```python
from build123d import *

# Parameters (mm, degrees)
SKETCH1_R           = 0.75
SKETCH1_R_2         = 0.5
BOSS_EXTRUDE1_DEPTH = 2


with BuildPart() as part:
    # Sketch1 → Boss-Extrude1 (new body)
    with BuildSketch(Plane.XY):
        with BuildLine():
            Line((0, 6), (0, 15))
            Line((0, 15), (4, 15))
            Line((4, 15), (4, 17))
            Line((4, 17), (0, 17))
            Line((0, 17), (0, 20.3))
            ThreePointArc((0, 20.3), (1.464466094, 23.835533906), (5, 25.3))
            Line((5, 25.3), (11.2, 25.3))
            ThreePointArc((11.2, 25.3), (14.735533906, 23.835533906), (16.2, 20.3))
            Line((16.2, 20.3), (16.2, 17))
            Line((16.2, 17), (12.2, 17))
            Line((12.2, 17), (12.2, 15))
            Line((12.2, 15), (16.2, 15))
            Line((16.2, 15), (16.2, 6))
            Line((16.2, 6), (12.2, 6))
            Line((12.2, 6), (12.2, 4))
            Line((12.2, 4), (16.2, 4))
            Line((16.2, 4), (16.2, 2))
            ThreePointArc((16.2, 2), (15.614213562, 0.585786438), (14.2, 0))
            Line((14.2, 0), (2, 0))
            ThreePointArc((2, 0), (0.585786438, 0.585786438), (0, 2))
            Line((0, 2), (0, 4))
            Line((0, 4), (4, 4))
            Line((4, 4), (4, 6))
            Line((4, 6), (0, 6))
        make_face()
        with Locations(Location((6, 12.5, 0), (0, 0, 180))):
            Circle(SKETCH1_R, mode=Mode.SUBTRACT)
        with Locations(Location((10.2, 12.5, 0), (0, 0, 180))):
            Circle(SKETCH1_R, mode=Mode.SUBTRACT)
        with Locations(Location((2.75, 19, 0), (0, 0, 180))):
            Circle(SKETCH1_R, mode=Mode.SUBTRACT)
        with Locations(Location((13.45, 19, 0), (0, 0, 180))):
            Circle(SKETCH1_R, mode=Mode.SUBTRACT)
        with Locations((10.2, 8.5)):
            Circle(SKETCH1_R, mode=Mode.SUBTRACT)
        with Locations((6, 8.5)):
            Circle(SKETCH1_R, mode=Mode.SUBTRACT)
        with Locations((3, 22.3)):
            Circle(SKETCH1_R_2, mode=Mode.SUBTRACT)
        with Locations((13.2, 22.3)):
            Circle(SKETCH1_R_2, mode=Mode.SUBTRACT)
        with Locations((13.45, 2)):
            Circle(SKETCH1_R, mode=Mode.SUBTRACT)
        with Locations((2.75, 2)):
            Circle(SKETCH1_R, mode=Mode.SUBTRACT)
    extrude(amount=BOSS_EXTRUDE1_DEPTH)


solid = part.part
```
The listing builds one solid part. Answer for the finished solid, in the listing's coordinates (mm). A direction names the side the tool comes from. Give positions to 0.01 mm unless a question says otherwise; leave off trailing zeros. Order: outer loops, then holes, each group sorted by start corner. A loop starts at its lowest first (then second) coordinate and runs counter-clockwise, first axis right, second up.
Item 1: The part is cut by section A-A, the plane x = 9.75. Give the vertices of the cut face in (y, z).
From the geometry:
outline: (0, 0) - (7.9, 0) - (7.9, 2) - (0, 2) - close; (9.1, 0) - (11.9, 0) - (11.9, 2) - (9.1, 2) - close; (13.1, 0) - (25.3, 0) - (25.3, 2) - (13.1, 2) - close
Item 2: The part is cut by section D-D, the plane x = 3. Give the vertices of the cut face in (y, z).
From the geometry:
outline: (0, 0) - (1.29, 0) - (1.29, 2) - (0, 2) - close; (2.71, 0) - (4, 0) - (4, 2) - (2.71, 2) - close; (6, 0) - (15, 0) - (15, 2) - (6, 2) - close; (17, 0) - (18.29, 0) - (18.29, 2) - (17, 2) - close; (19.71, 0) - (21.8, 0) - (21.8, 2) - (19.71, 2) - close; (22.8, 0) - (24.88, 0) - (24.88, 2) - (22.8, 2) - close
Item 3: For a pull along X with two mould halves and no side action, classify faces 3 (the face through (16.2, 19, 1)), 4 (the face through (2, 4, 1)), 5 (the face through (10.915, 8.725, 0.986)), 6 (the face through (4, 5, 1)) as pulls with the +X half, pulls with the -X half, needs draft (parallel to the pull), parting line crosses it, or undercut.
From the geometry:
face 3: pulls with the +X half
face 4: needs draft
face 5: undercut
face 6: pulls with the -X half
Item 4: Which of the six approach directions +Z, -Z, +X, -X, +Y, -Y give full straight-line access (tool end or side, diameter ignored) to faces 1 (the face through (14, 15, 1)), 2 (the face through (1.43, 23.8, 0.99))?
From the geometry:
face 1: +Z, -Z, +X
face 2: +Z, -Z, -X, +Y
Item 5: Find the intervals of material crossed by probe 1 along Y at (x, z) = (6, 0.85); probe 2 along X at (y, z) = (12.5, 1.45); probe 3 along X at (y, z) = (19, 1.1), in increasing order.
From the geometry:
probe 1: y = 0 to 7.75, 9.25 to 11.75, 13.25 to 25.3
probe 2: x = 0 to 5.25, 6.75 to 9.45, 10.95 to 16.2
probe 3: x = 0 to 2, 3.5 to 12.7, 14.2 to 16.2
Item 6: The part is cut by section B-B, the plane z = 1.05. Count the separate pieces of the cut face and the enclosed holes in it, and give its area (3 significant figures).
From the geometry:
separate pieces: 1
enclosed holes: 10
area: 350 mm2
Item 7: The part is cut by section C-C, the plane y = 2.25. Give the vertices of the cut face in (x, z).
From the geometry:
outline: (0, 0) - (2.04, 0) - (2.04, 2) - (0, 2) - close; (3.46, 0) - (12.74, 0) - (12.74, 2) - (3.46, 2) - close; (14.16, 0) - (16.2, 0) - (16.2, 2) - (14.16, 2) - close
Item 8: Given pin 1 Ø0.6 at (y, z) = (16, 1.5) entering from -X; pin 2 Ø0.6 at (x, z) = (13.5, 1) entering from +Y, each flat-ended and moving along its own axis, determine where each tip first touches the part or whether it passes through.
From the geometry:
pin 1: stops at x = 4
pin 2: stops at y = 24.88
